Answer from the drawing. Dimensions are ordinates in mm from the lowest x, y and z of the part. A direction names the side the tool comes from. Give positions to 0.01 mm unless a question says otherwise; leave off trailing zeros. Loops run counter-clockwise (first coordinate to the right, second up) from the corner with the lowest first, then second, coordinate; pieces in that order, holes last. Notation, with made-up numbers: M -6,-29 L 21,-29 A12 ccw 21,-20 Z; hole C -28.5,77 d11. An arc over 180 degrees is marked long. Use a Markdown table: item, result.
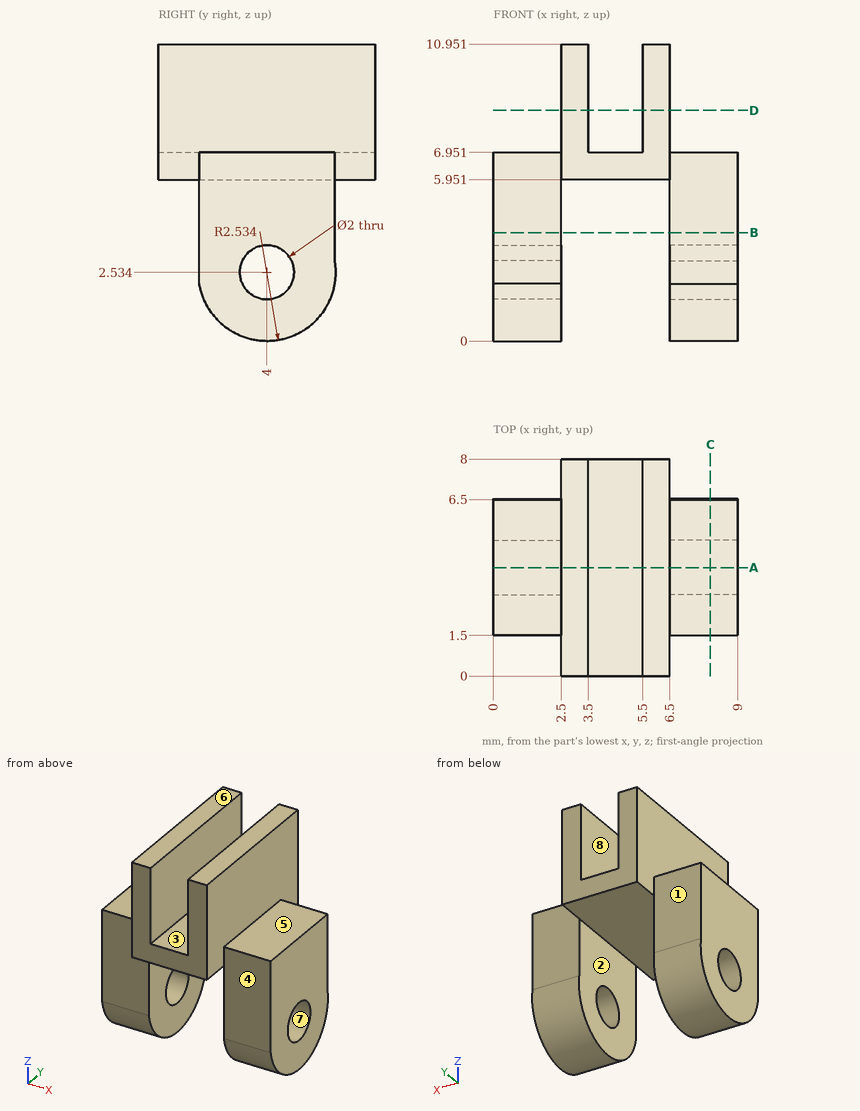
(1) Given P1, Ø2, axis at x = 8.5, y = 4.5, coming from the +Z side; P2, Ø1.2, axis at y = 4, z = 2.53, coming from the -X side; P3, Ø4, axis at x = 3, y = 2, coming from the -Z side; P4, Ø1.2, axis at x = 7.5, z = 5.5, coming from the +Y side, each flat-ended and moving along its own axis, determine where each tip first touches the part or whether it passes through.
Entries:
| item | result |
|---|---|
| P1 | stops at z = 6.95 |
| P2 | passes through |
| P3 | stops at z = 0 |
| P4 | stops at y = 6.5 |
(2) Consider probe 1 along X at (y, z) = (4.5, 5); probe 2 along X at (y, z) = (6, 7.75); probe 3 along Y at (x, z) = (1, 6). Determine where each line is inside the solid, lowest interval first. Write a range as [from, to].
Entries:
| item | result |
|---|---|
| probe 1 | x = [0, 2.5], [6.5, 9] |
| probe 2 | x = [2.5, 3.5], [5.5, 6.5] |
| probe 3 | y = [1.5, 6.5] |
(3) A cutting plane is placed at B-B (z = 4). Write down the section's boundary in (x, y).
Entries:
| item | result |
|---|---|
| outline | M 0,1.5 L 2.5,1.5 L 2.5,6.5 L 0,6.5 Z; M 6.5,1.5 L 9,1.5 L 9,6.5 L 6.5,6.5 Z |
(4) A cutting plane is placed at C-C (x = 8). Write down the section's boundary in (y, z) (1 decimal).
Entries:
| item | result |
|---|---|
| outline | M 1.5,2.1 A2.5 ccw 6.5,3 L 6.5,7 L 1.5,7 Z; hole C 4,2.5 d2 |
(5) A cutting plane is placed at D-D (z = 8.5). Write down the section's boundary in (x, y), and give its area (3 significant figures).
Entries:
| item | result |
|---|---|
| outline | M 2.5,0 L 3.5,0 L 3.5,8 L 2.5,8 Z; M 5.5,0 L 6.5,0 L 6.5,8 L 5.5,8 Z |
| area | 16.0 mm² |
(6) Which of the six approach directions +Z, -Z, +X, -X, +Y, -Y give full straight-line access (tool end or side, diameter ignored) to the marked faces 1, 2, 3, 4 and 5?
Entries:
| item | result |
|---|---|
| face 1 | +Z, -X, +Y |
| face 2 | -Z, +Y, -Y |
| face 3 | +Z, +Y, -Y |
| face 4 | +Z, -Z, +X, -Y |
| face 5 | +Z, +X, +Y, -Y |
(7) The mould has two halves that part along Z. Classify the marked faces 6, 7 and 8: released by +Z, released by -Z, zero draft, split by the parting line, or undercut.
Entries:
| item | result |
|---|---|
| face 6 | released by +Z |
| face 7 | undercut |
| face 8 | zero draft |
(8) A cutting plane is placed at A-A (y = 4). Write down the section's boundary in (x, z) (1 decimal).
Entries:
| item | result |
|---|---|
| outline | M 0,0 L 2.5,0 L 2.5,1.5 L 0,1.5 Z; M 0,3.5 L 2.5,3.5 L 2.5,6 L 6.5,6 L 6.5,3.5 L 9,3.5 L 9,7 L 6.5,7 L 6.5,11 L 5.5,11 L 5.5,7 L 3.5,7 L 3.5,11 L 2.5,11 L 2.5,7 L 0,7 Z; M 6.5,0 L 9,0 L 9,1.5 L 6.5,1.5 Z |
